Check sheet for the modelled part. Datum: model origin and axes. Units: mm. Face numbers are marked on the shaded views. Give positions to 0.01 mm unless a question says otherwise; leave off trailing zeros. Order: outer loops, then holes, each group sorted by start corner. A loop starts at its lowest first (then second) coordinate and runs counter-clockwise, first axis right, second up.
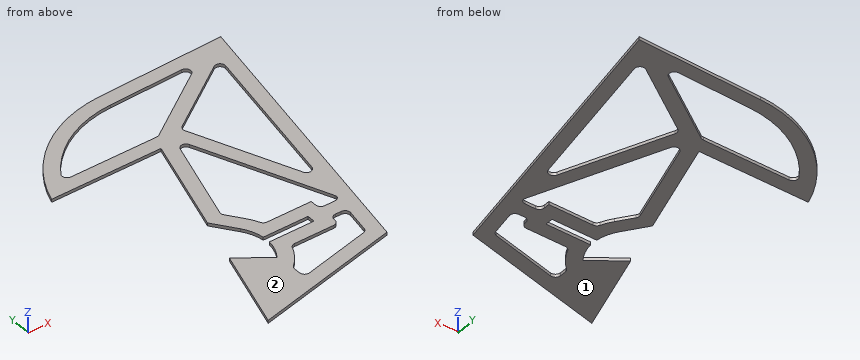
from build123d import *

# Parameters (mm, degrees)
BOSS_EXTRUDE2_DEPTH = 0.762
CUT_EXTRUDE1_DEPTH  = 2.54
FILLET1_R           = 1.27
FILLET2_R           = 1.27


with BuildPart() as part:
    # Sketch1 → Boss-Extrude2 (new body)
    with BuildSketch(Plane.XY):
        with BuildLine():
            Line((-17.038837989, 37.195), (-24.885307058, 11.67932501))
            Line((-24.885307058, 11.67932501), (-20.799118841, 6.0325))
            ThreePointArc((-20.799118841, 6.0325), (-19.511844062, 3.642975475), (-18.894118841, 1))
            Line((-18.894118841, 1), (-7.464118841, 1))
            Line((-7.464118841, 1), (-7.464118841, -1))
            Line((-7.464118841, -1), (-18.894118841, -1))
            ThreePointArc((-18.894118841, -1), (-19.511844062, -3.642975475), (-20.799118841, -6.0325))
            Line((-20.799118841, -6.0325), (-28.596784868, -0.38990775))
            Line((-28.596784868, -0.38990775), (-35.143553898, -21.67913088))
            Line((-35.143553898, -21.67913088), (1.940239682, -12.938292607))
            Line((1.940239682, -12.938292607), (15.418184296, 59.478146197))
            Line((15.418184296, 59.478146197), (-16.317685222, 58.531))
            ThreePointArc((-16.317685222, 58.531), (-34.007299879, 52.375275454), (-44.978837989, 37.195))
            Line((-44.978837989, 37.195), (-17.038837989, 37.195))
        make_face()
    extrude(amount=-BOSS_EXTRUDE2_DEPTH)

    # Sketch2 → Cut-Extrude1 (cut)
    with BuildSketch(Plane(origin=(0, 0, -0.762), x_dir=(-1, 0, 0), z_dir=(0, 0, -1))):
        Polygon((9.959013349, 39.898911244), (-10.811031118, 54.15844292), (-2.469426207, 9.339344835), align=None)
        with BuildLine():
            Line((16.211604848, 54.976582614), (-6.716661044, 55.660868886))
            Line((-6.716661044, 55.660868886), (15.000646844, 40.751))
            Line((15.000646844, 40.751), (39.552648945, 40.751))
            ThreePointArc((39.552648945, 40.751), (29.764823586, 50.952881409), (16.211604848, 54.976582614))
        make_face()
        with BuildLine():
            Line((13.163553789, 37.698855968), (12.959946202, 37.838641361))
            Line((12.959946202, 37.838641361), (-1.264200274, 2.863715758))
            Line((-1.264200274, 2.863715758), (-1.0621299, 1.778))
            Line((-1.0621299, 1.778), (3.908118841, 1.778))
            Line((3.908118841, 1.778), (3.908118841, 4.556))
            Line((3.908118841, 4.556), (16.060442021, 4.556))
            ThreePointArc((16.060442021, 4.556), (16.85953464, 6.404305379), (17.918263947, 8.117160903))
            Line((17.918263947, 8.117160903), (20.965443108, 12.328148402))
            Line((20.965443108, 12.328148402), (13.163553789, 37.698855968))
        make_face()
        with BuildLine():
            Line((3.908118841, -1.778), (-0.400297147, -1.778))
            Line((-0.400297147, -1.778), (1.131614758, -10.008899288))
            Line((1.131614758, -10.008899288), (20.37916729, -14.545645063))
            Line((20.37916729, -14.545645063), (20.37916729, -10.725757063))
            ThreePointArc((20.37916729, -10.725757063), (17.792273547, -7.940143054), (16.060442021, -4.556))
            Line((16.060442021, -4.556), (3.908118841, -4.556))
            Line((3.908118841, -4.556), (3.908118841, -1.778))
        make_face()
    extrude(amount=-CUT_EXTRUDE1_DEPTH, mode=Mode.SUBTRACT)

    # Fillet1
    # the kernel refuses this fillet: 1.27 mm, written as the material it adds along each edge
    with BuildSketch(Plane(origin=(-39.552648945, 40.751, -0.762), x_dir=(0.5208478104072599, 0.8536495524475856, 0), z_dir=(0, 0, 1))) as fillet1_piece_1:
        with BuildLine():
            CenterArc((2.261930285, -1.268884618), FILLET1_R, 87.598517958, 123.790620182)
            Line((1.177795353, -1.930361337), (0, 0))
            ThreePointArc((0, 0), (1.157572593, 0.024262667), (2.315145186, 0))
        make_face()
    extrude(amount=0.762)
    with BuildSketch(Plane(origin=(-15.000646844, 40.751, -0.762), x_dir=(-1, 0, 0), z_dir=(0, 0, 1))) as fillet1_piece_2:
        with BuildLine():
            CenterArc((FILLET1_R * 0.310233467687, -FILLET1_R), FILLET1_R, 90, 34.471278604)
            Line((-FILLET1_R * 0.2557595777, -FILLET1_R * 0.175589985157), (0, 0))
            Line((0, 0), (FILLET1_R * 0.310233467687, 0))
        make_face()
    extrude(amount=0.762)
    with BuildSketch(Plane(origin=(6.716661044, 55.660868886, -0.762), x_dir=(-0.9995549454578584, -0.029831376279645935, 0), z_dir=(0, 0, 1))) as fillet1_piece_3:
        with BuildLine():
            CenterArc((FILLET1_R * 3.40189361791, FILLET1_R), FILLET1_R, 122.761813037, 147.238186963)
            Line((FILLET1_R * 2.86074575566, FILLET1_R * 1.84092745893), (0, 0))
            Line((0, 0), (FILLET1_R * 3.40189361791, 0))
        make_face()
    extrude(amount=0.762)
    with BuildSketch(Plane(origin=(-16.060442021, -4.556, -0.762), x_dir=(1, 0, 0), z_dir=(0, 0, 1))) as fillet1_piece_4:
        with BuildLine():
            CenterArc((0.873205275, -1.27), FILLET1_R, 90, 67.330529822)
            ThreePointArc((-0.298679081, -0.780523691), (-0.143449411, -0.392515792), (0, 0))
            Line((0, 0), (0.873205275, 0))
        make_face()
    extrude(amount=0.762)
    with BuildSketch(Plane(origin=(-20.37916729, -10.725757063, -0.762), x_dir=(0.7616549867095258, 0.6479827784906881, 0), z_dir=(0, 0, 1))) as fillet1_piece_5:
        with BuildLine():
            CenterArc((0.587183206, -1.269738966), FILLET1_R, 91.161693546, 48.448622341)
            Line((-0.380118627, -0.446800838), (0, 0))
            ThreePointArc((0, 0), (0.28071762, -0.002845925), (0.561435241, 0))
        make_face()
    extrude(amount=0.762)
    with BuildSketch(Plane(origin=(-20.37916729, -14.545645063, -0.762), x_dir=(0, 1, 0), z_dir=(0, 0, 1))) as fillet1_piece_6:
        with BuildLine():
            CenterArc((FILLET1_R * 1.26310805209, -FILLET1_R), FILLET1_R, 90, 103.262828677)
            Line((FILLET1_R * 0.289780136608, -FILLET1_R * 1.22941832738), (0, 0))
            Line((0, 0), (FILLET1_R * 1.26310805209, 0))
        make_face()
    extrude(amount=0.762)
    with BuildSketch(Plane(origin=(-1.131614758, -10.008899288, -0.762), x_dir=(-0.9733279154855742, -0.22941832737710197, 0), z_dir=(0, 0, 1))) as fillet1_piece_7:
        with BuildLine():
            CenterArc((FILLET1_R * 0.651818100075, -FILLET1_R), FILLET1_R, 90, 66.194073158)
            Line((-FILLET1_R * 0.263099818984, -FILLET1_R * 0.596360059726), (0, 0))
            Line((0, 0), (FILLET1_R * 0.651818100075, 0))
        make_face()
    extrude(amount=0.762)
    with BuildSketch(Plane(origin=(0.400297147, -1.778, -0.762), x_dir=(-1, 0, 0), z_dir=(0, 0, 1))) as fillet1_piece_8:
        with BuildLine():
            CenterArc((FILLET1_R * 1.20328955763, FILLET1_R), FILLET1_R, 169.456901836, 100.543098164)
            Line((FILLET1_R * 0.220172006676, FILLET1_R * 1.182975083), (0, 0))
            Line((0, 0), (FILLET1_R * 1.20328955763, 0))
        make_face()
    extrude(amount=0.762)
    with BuildSketch(Plane(origin=(-3.908118841, -1.778, -0.762), x_dir=(1, 0, 0), z_dir=(0, 0, 1)), Plane(origin=(-3.908118841, 1.778, -0.762), x_dir=(0, 1, 0), z_dir=(0, 0, 1))) as fillet1_piece_9:
        with BuildLine():
            CenterArc((FILLET1_R, -FILLET1_R), FILLET1_R, 90, 90)
            Line((0, -FILLET1_R), (0, 0))
            Line((0, 0), (FILLET1_R, 0))
        make_face()
    extrude(amount=0.762)
    with BuildSketch(Plane(origin=(10.811031118, 54.15844292, -0.762), x_dir=(-0.8244100148431994, -0.5659930453868101, 0), z_dir=(0, 0, 1))) as fillet1_piece_10:
        with BuildLine():
            CenterArc((FILLET1_R * 2.41507052303, FILLET1_R), FILLET1_R, 134.985623232, 135.014376768)
            Line((FILLET1_R * 1.7081411927, FILLET1_R * 1.70728418753), (0, 0))
            Line((0, 0), (FILLET1_R * 2.41507052303, 0))
        make_face()
    extrude(amount=0.762)
    with BuildSketch(Plane(origin=(-9.959013349, 39.898911244, -0.762), x_dir=(0.824410014843199, 0.5659930453868107, 0), z_dir=(0, 0, 1))) as fillet1_piece_11:
        with BuildLine():
            CenterArc((FILLET1_R * 0.804884205906, -FILLET1_R), FILLET1_R, 90, 77.660077981)
            Line((-FILLET1_R * 0.172012698042, -FILLET1_R * 0.786288888787), (0, 0))
            Line((0, 0), (FILLET1_R * 0.804884205906, 0))
        make_face()
    extrude(amount=0.762)
    with BuildSketch(Plane(origin=(2.469426207, 9.339344835, -0.762), x_dir=(-0.37673127332714895, 0.9263225937530105, 0), z_dir=(0, 0, 1))) as fillet1_piece_12:
        with BuildLine():
            CenterArc((FILLET1_R * 3.41150341271, -FILLET1_R), FILLET1_R, 90, 147.325545251)
            Line((FILLET1_R * 2.87163833244, -FILLET1_R * 1.84175156376), (0, 0))
            Line((0, 0), (FILLET1_R * 3.41150341271, 0))
        make_face()
    extrude(amount=0.762)
    with BuildSketch(Plane(origin=(-16.060442021, 4.556, -0.762), x_dir=(-0.35739171022603367, 0.9339545842607717, 0), z_dir=(0, 0, 1))) as fillet1_piece_13:
        with BuildLine():
            CenterArc((0.874045995, -1.269421541), FILLET1_R, 91.729372014, 67.330529822)
            Line((-0.312076327, -0.815534069), (0, 0))
            ThreePointArc((0, 0), (0.417859553, -0.006306655), (0.835719106, 0))
        make_face()
    extrude(amount=0.762)
    with BuildSketch(Plane(origin=(1.0621299, 1.778, -0.762), x_dir=(-1, 0, 0), z_dir=(0, 0, 1))) as fillet1_piece_14:
        with BuildLine():
            CenterArc((FILLET1_R * 0.831055163452, -FILLET1_R), FILLET1_R, 90, 79.456901836)
            Line((-FILLET1_R * 0.152062387507, -FILLET1_R * 0.817024917004), (0, 0))
            Line((0, 0), (FILLET1_R * 0.831055163452, 0))
        make_face()
    extrude(amount=0.762)
    with BuildSketch(Plane(origin=(1.264200274, 2.863715758, -0.762), x_dir=(-0.18297508299575613, -0.9831175509585292, 0), z_dir=(0, 0, 1))) as fillet1_piece_15:
        with BuildLine():
            CenterArc((FILLET1_R * 0.293125897595, -FILLET1_R), FILLET1_R, 90, 32.674454749)
            Line((-FILLET1_R * 0.24673918268, -FILLET1_R * 0.158248436236), (0, 0))
            Line((0, 0), (FILLET1_R * 0.293125897595, 0))
        make_face()
    extrude(amount=0.762)
    with BuildSketch(Plane(origin=(-13.163553789, 37.698855968, -0.762), x_dir=(0.8244100148432169, 0.5659930453867846, 0), z_dir=(0, 0, 1))) as fillet1_piece_16:
        with BuildLine():
            CenterArc((0.466869862, -1.250818003), FILLET1_R, 99.970819011, 28.464420859)
            Line((-0.322599825, -0.256012688), (0, 0))
            Line((0, 0), (0.246973695, 0))
        make_face()
    extrude(amount=0.762)
    with BuildSketch(Plane(origin=(-20.965443108, 12.328148402, -0.762), x_dir=(0.29393158388003876, 0.9558264612353917, 0), z_dir=(0, 0, 1))) as fillet1_piece_17:
        with BuildLine():
            CenterArc((FILLET1_R * 0.49840674513, -FILLET1_R), FILLET1_R, 90, 52.983950443)
            Line((-FILLET1_R * 0.300060154598, -FILLET1_R * 0.397961288587), (0, 0))
            Line((0, 0), (FILLET1_R * 0.49840674513, 0))
        make_face()
    extrude(amount=0.762)
    # the kernel refuses this fillet: 1.27 mm, written as the material it takes off along each edge
    with BuildSketch(Plane(origin=(-3.908118841, -4.556, -3.937), x_dir=(0, 1, 0), z_dir=(0, 0, 1))) as fillet1_2_piece_1:
        with BuildLine():
            CenterArc((FILLET1_R, FILLET1_R), FILLET1_R, 180, 90)
            Line((0, FILLET1_R), (0, 0))
            Line((0, 0), (FILLET1_R, 0))
        make_face()
    extrude(amount=7.112, mode=Mode.SUBTRACT)

    # Fillet2
    # the kernel refuses this fillet: 1.27 mm, written as the material it adds along each edge
    with BuildSketch(Plane(origin=(-12.959946202, 37.838641361, -0.762), x_dir=(-0.33704949641536375, -0.9414869287282484, 0), z_dir=(0, 0, 1))) as fillet2_piece_1:
        with BuildLine():
            CenterArc((3.321849705, 1.268688867), FILLET2_R, 131.828571636, 140.775161889)
            Line((2.474881455, 2.215021147), (2.390184631, 2.309654375))
            Line((2.390184631, 2.309654375), (-0.084696825, 0.094633228))
            Line((-0.084696825, 0.094633228), (-0.055395427, -0.114281874))
            ThreePointArc((-0.055395427, -0.114281874), (0.617417306, -0.252739018), (3.385312737, -0.126868887))
            Line((3.385312737, -0.126868887), (3.37954337, 0))
        make_face()
    extrude(amount=0.762)


solid = part.part
1) Section check C-C, the plane x = 6.5. Record the cut outline in (y, z), then the cut area to 3 significant figures.
Recorded:
outline: (11.56, -0.76) - (31, -0.76) - (31, 0) - (11.56, 0) - close; (51.2, -0.76) - (59.21, -0.76) - (59.21, 0) - (51.2, 0) - close
area: 20.9 mm2
2) Section check B-B, the plane y = 22. Record the cut outline in (x, z), then the cut area to 3 significant figures.
Recorded:
outline: (-21.71, -0.76) - (-17.99, -0.76) - (-17.99, 0) - (-21.71, 0) - close; (-6.52, -0.76) - (-2.68, -0.76) - (-2.68, 0) - (-6.52, 0) - close; (4.83, -0.76) - (8.44, -0.76) - (8.44, 0) - (4.83, 0) - close
area: 8.52 mm2
3) Material ranges on L1, parallel to X at y = 30, z = -0.7; L2, parallel to Y at x = -2, z = -0.55; L3, parallel to Y at x = -1.5, z = -0.3, recorded low to high.
Recorded:
L1: x = -19.25 to -15.53, -9.77 to -5.93, 6.31 to 9.93
L2: y = -13.87 to -10.21, -1.78 to 1.78, 10.89 to 20.33, 45.36 to 49.68, 55.4 to 58.96
L3: y = -13.75 to -10, -1.78 to 1.78, 9.66 to 19.1, 45.71 to 50.02, 55.42 to 58.97
4) Section check A-A, the plane x = -30. Record the cut outline in (y, z) (3 decimals).
Recorded:
outline: (-20.467, -0.762) - (-4.953, -0.762) - (-4.953, 0) - (-20.467, 0) - close; (37.195, -0.762) - (40.751, -0.762) - (40.751, 0) - (37.195, 0) - close; (50.808, -0.762) - (54.909, -0.762) - (54.909, 0) - (50.808, 0) - close
5) Section check D-D, the plane z = -0.35. State how many separate pieces and enclosed holes the cut face has, then the cut area to 3 significant figures.
Recorded:
separate pieces: 1
enclosed holes: 4
area: 1,360 mm2
6) Depth check by flat-ended pin: pin 1 Ø6 at (x, y) = (-11.5, 18.5) entering from +Z; pin 2 Ø6 at (x, y) = (-30, -4.5) entering from -Z. Enter the tip coordinate at first touch or a pass-through.
Recorded:
pin 1: passes through
pin 2: stops at z = -0.76
7) Draft check along Z on the marked faces 1 and 2. Enter one of: +Z half, -Z half, draft (parallel to the pull), parting line (faces both ways), or undercut.
Recorded:
face 1: -Z half
face 2: +Z half
